The listing builds one solid part. Answer for the finished solid, in the listing's coordinates (mm). Round coordinates to 2 decimals unless told otherwise and drop trailing zeros. Write each loop counter-clockwise with the first axis right and the second up, starting at its lowest first coordinate (ties: lowest second). Pieces come first, ordered by that corner, then holes.
Item 1: Find section B-B on y = 72.5. Give the vertices of the cut face in (x, z), then the cut area to 3 significant figures.
Item 2: For a pull along Y with two mould halves and no side action, classify faces 1 (the face through (-62.963, 31.665, 22.442)), 2 (the face through (-92, 27.784, 23)), 3 (the face through (-91, 54, 20)) as +Y half, -Y half, draft (parallel to the pull), parting line (faces both ways), or undercut.
Item 3: Each of these flat-tipped pins is pushed along its axis until it touches: pin 1 (3.5 mm diameter, centred on x = -115.905, y = 75.538, fed in from +Z); pin 2 (3 mm diameter, centred on x = -69, z = 24, fed in from -Y); pin 3 (8 mm diameter, centred on x = -100.5, y = 50.5, fed in from +Z). Where does it stop, or does it pass through?
Item 4: Find the intervals of material crossed by probe 1 along X at (y, z) = (75.44, 22.95); probe 2 along Y at (x, z) = (-63, 21); probe 3 along Y at (x, z) = (-133, 25.5), in increasing order.
```python
from build123d import *

# Parameters (mm, degrees)
BOSS_EXTRUDE1_START = 20
BOSS_EXTRUDE1_DEPTH = 2
BOSS_EXTRUDE2_DEPTH = 52.64
SKETCH5_R           = 1.1
CUT_EXTRUDE2_DEPTH  = 19.64
SKETCH5_5_R         = 1.1
CUT_EXTRUDE3_DEPTH  = 19.64
SKETCH5_6_R         = 1.1
CUT_EXTRUDE4_DEPTH  = 19.64
SKETCH5_7_R         = 1.1
CUT_EXTRUDE5_DEPTH  = 19.64
FILLET1_R           = 1
FILLET2_R           = 1


with BuildPart() as part:
    # Sketch2 → Boss-Extrude1 (new body)
    with BuildSketch(Plane.XY.offset(BOSS_EXTRUDE1_START)):
        Polygon((-121.572, 80.424), (-41.572, 80.424), (-41.572, 27.78), (-141.572, 27.78), (-141.572, 80.424), align=None)
    extrude(amount=BOSS_EXTRUDE1_DEPTH)

    # Sketch3 → Boss-Extrude2 (add)
    with BuildSketch(Plane(origin=(0, 80.424, 0), x_dir=(1, 0, 0), z_dir=(0, 1, 0))):
        with BuildLine():
            Line((-41.572, -28), (-41.572, -22))
            Line((-41.572, -22), (-141.572, -22))
            Line((-141.572, -22), (-141.572, -28))
            ThreePointArc((-141.572, -28), (-91.572, -23.213616387), (-41.572, -28))
        make_face()
    extrude(amount=-BOSS_EXTRUDE2_DEPTH)

    # Sketch5 → Cut-Extrude2 (cut)
    with BuildSketch(Plane(origin=(0, 0, 20), x_dir=(-1, 0, 0), z_dir=(0, 0, -1))):
        with Locations((62.455, 32.641)):
            Circle(SKETCH5_R)
    extrude(amount=-CUT_EXTRUDE2_DEPTH, mode=Mode.SUBTRACT)

    # Sketch5<5> → Cut-Extrude3 (cut)
    with BuildSketch(Plane(origin=(0, 0, 20), x_dir=(-1, 0, 0), z_dir=(0, 0, -1))):
        with Locations((62.836, 75.44)):
            Circle(SKETCH5_5_R)
    extrude(amount=-CUT_EXTRUDE3_DEPTH, mode=Mode.SUBTRACT)

    # Sketch5<6> → Cut-Extrude4 (cut)
    with BuildSketch(Plane(origin=(0, 0, 20), x_dir=(-1, 0, 0), z_dir=(0, 0, -1))):
        with Locations((115.905, 75.538)):
            Circle(SKETCH5_6_R)
    extrude(amount=-CUT_EXTRUDE4_DEPTH, mode=Mode.SUBTRACT)

    # Sketch5<7> → Cut-Extrude5 (cut)
    with BuildSketch(Plane(origin=(0, 0, 20), x_dir=(-1, 0, 0), z_dir=(0, 0, -1))):
        with Locations((117.094, 33.147)):
            Circle(SKETCH5_7_R)
    extrude(amount=-CUT_EXTRUDE5_DEPTH, mode=Mode.SUBTRACT)

    # Fillet1
    fillet1_edges = [part.edges().sort_by_distance(p)[0] for p in [
        (-41.572, 54.104, 28),
    ]]
    fillet(fillet1_edges, radius=FILLET1_R)

    # Fillet2
    fillet2_edges = [part.edges().sort_by_distance(p)[0] for p in [
        (-141.572, 54.104, 28),
    ]]
    fillet(fillet2_edges, radius=FILLET2_R)


solid = part.part
```
Check values:
1. outline: (-141.57, 20) - (-41.57, 20) - (-41.57, 26.79) arc R1 ccw to (-42.76, 27.77) arc R263.55 cw to (-140.39, 27.77) arc R1 ccw to (-141.57, 26.79) - close
1. area: 480 mm2
2. face 1: undercut
2. face 2: -Y half
2. face 3: draft
3. pin 1: stops at z = 24.51
3. pin 2: stops at y = 27.78
3. pin 3: stops at z = 23.53
4. probe 1: x = -141.57 to -117, -114.81 to -63.94, -61.74 to -41.57
4. probe 2: y = 27.78 to 31.69, 33.6 to 74.35, 76.53 to 80.42
4. probe 3: y = 27.78 to 80.42
